Input: dimensioned drawing with shaded views. Units: mm. Origin: part minimum x, y, z. Give positions to 0.01 mm unless a question says otherwise; leave off trailing zeros. Order: outer loops, then holes, each group sorted by start corner. A loop starts at its lowest first (then second) coordinate and runs counter-clockwise, first axis right, second up. Notation, with made-up numbers: (-26, 74) - (-15, 74) arc R19 cw to (-15, 98) - close; hole circle Ø2 at (0.5, -18). An arc over 180 degrees is marked (long way). Use a Markdown table: item, result.
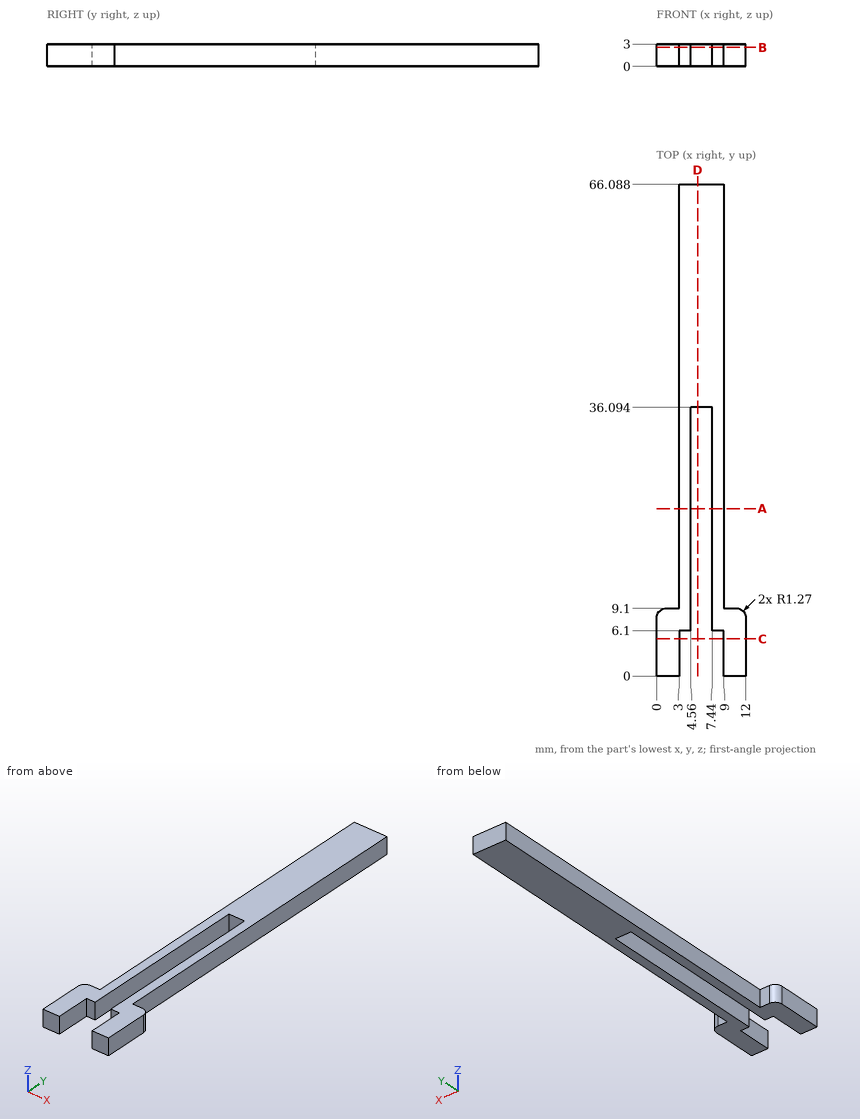
1. Section query C-C (y = 5). Return loops of the section in (x, z).
Response:
| item | result |
|---|---|
| outline | (0, 0) - (3, 0) - (3, 3) - (0, 3) - close; (9, 0) - (12, 0) - (12, 3) - (9, 3) - close |
2. Material intervals for line 1 along X through (y, z) = (31, 1.45); line 2 along X through (y, z) = (7, 2.2); line 3 along X through (y, z) = (47.5, 2.1), sorted ascending.
Response:
| item | result |
|---|---|
| line 1 | x = 3 to 4.56, 7.44 to 9 |
| line 2 | x = 0 to 4.56, 7.44 to 12 |
| line 3 | x = 3 to 9 |
3. Pin query (flat end, axial travel): pin 1 (0.9 mm diameter, centred on y = 31.5, z = 1, fed in from -X); pin 2 (1.5 mm diameter, centred on y = 27, z = 1.5, fed in from +X); pin 3 (0.9 mm diameter, centred on x = 9.5, z = 1, fed in from +Y). Return the tip coordinate at first contact, or that it passes through.
Response:
| item | result |
|---|---|
| pin 1 | stops at x = 3 |
| pin 2 | stops at x = 9 |
| pin 3 | stops at y = 9.1 |
4. Section query B-B (z = 2.55). Return loops of the section in (x, y).
Response:
| item | result |
|---|---|
| outline | (0, 0) - (3, 0) - (3, 6.1) - (4.56, 6.1) - (4.56, 36.09) - (7.44, 36.09) - (7.44, 6.1) - (9, 6.1) - (9, 0) - (12, 0) - (12, 7.83) arc R1.27 ccw to (10.73, 9.1) - (9, 9.1) - (9, 66.09) - (3, 66.09) - (3, 9.1) - (1.27, 9.1) arc R1.27 ccw to (0, 7.83) - close |
5. Section query D-D (x = 5.5). Return loops of the section in (y, z), then the cut area to 3 significant figures.
Response:
| item | result |
|---|---|
| outline | (36.09, 0) - (66.09, 0) - (66.09, 3) - (36.09, 3) - close |
| area | 90.0 mm^2 |
6. Section query A-A (y = 22.5). Return loops of the section in (x, z).
Response:
| item | result |
|---|---|
| outline | (3, 0) - (4.56, 0) - (4.56, 3) - (3, 3) - close; (7.44, 0) - (9, 0) - (9, 3) - (7.44, 3) - close |
